from build123d import *

# Parameters (mm, degrees)
F1_DEPTH = 52
F2_DEPTH = 22
F0_R     = 9
F3_DEPTH = 34


with BuildPart() as f1:
    # F0 (on Front) → F1 (new body)
    with BuildSketch(Plane.XZ):
        with BuildLine():
            Line((14, 34), (-54, 34))
            ThreePointArc((-54, 34), (-63.150826, 32.745418), (-71.62633, 29.074258))
            ThreePointArc((-71.62633, 29.074258), (-86.745418, -9.150826), (-54, -34))
            Line((-54, -34), (54, -34))
            ThreePointArc((54, -34), (85.140624, -13.647768), (79, 23.043437))
            ThreePointArc((79, 23.043437), (67.647768, 31.140624), (54, 34))
            Line((54, 34), (27.266499, 34))
            Line((27.266499, 34), (14, 34))
        make_face()
        with BuildLine():
            ThreePointArc((-54, -15), (-69, 0), (-54, 15))
            Line((-54, 15), (54, 15))
            ThreePointArc((54, 15), (69, 0), (54, -15))
            Line((54, -15), (-54, -15))
        make_face(mode=Mode.SUBTRACT)
    extrude(amount=F1_DEPTH)

    # F0 (on Front) → F2 (join)
    with BuildSketch(Plane.XZ):
        with BuildLine():
            ThreePointArc((-71.62633, 29.074258), (-63.150826, 32.745418), (-54, 34))
            Line((-54, 34), (14, 34))
            ThreePointArc((14, 34), (24.606602, 38.393398), (29, 49))
            Line((29, 49), (29, 76))
            ThreePointArc((29, 76), (32.216825, 88.267571), (41.039463, 97.378131))
            Line((41.039463, 97.378131), (-71.62633, 29.074258))
        make_face()
    extrude(amount=F2_DEPTH)

    # F0 (on Front) → F3 (join)
    with BuildSketch(Plane.XZ):
        with BuildLine():
            ThreePointArc((29, 49), (24.606602, 38.393398), (14, 34))
            Line((14, 34), (27.266499, 34))
            Line((27.266499, 34), (54, 34))
            ThreePointArc((54, 34), (67.647768, 31.140624), (79, 23.043437))
            Line((79, 23.043437), (79, 76))
            ThreePointArc((79, 76), (54, 51), (29, 76))
            Line((29, 76), (29, 49))
        make_face()
        with BuildLine():
            ThreePointArc((79, 76), (66.267571, 97.783175), (41.039463, 97.378131))
            ThreePointArc((41.039463, 97.378131), (32.216825, 88.267571), (29, 76))
            ThreePointArc((29, 76), (54, 51), (79, 76))
        make_face()
        with Locations((54, 76)):
            Circle(F0_R, mode=Mode.SUBTRACT)
    extrude(amount=F3_DEPTH)


solid = f1.part
Geometry: final body of the model. Coordinates: model frame, mm. A direction names the side the tool comes from. Coordinates: 2 decimals unless noted, no trailing zeros. Write each loop counter-clockwise with the first axis right and the second up, starting at its lowest first coordinate (ties: lowest second). Pieces come first, ordered by that corner, then holes. Notation, with made-up numbers: (32, 82) - (58, 82) arc R28 cw to (58, 116) - close; hole circle Ø6 at (-16, -28). An arc over 180 degrees is marked (long way). Return JSON: item names as keys, results as strings.
Item 1: Pull-direction query (Z, two-part tool) for faces 5 (the face through (-1, -26, 15)), 6 (the face through (-3, -22, 51)), 7 (the face through (-1, -26, -34)); classes: +Z half, -Z half, draft (parallel to the pull), parting line (faces both ways), or undercut.
Completed:
{"face 5": "undercut", "face 6": "draft", "face 7": "-Z half"}
Item 2: Section query D-D (x = 72.5). Output: boundary loops of the cut face in (y, z), and give its area (3 significant figures).
Completed:
{"outline": "(-52, -28.53) - (0, -28.53) - (0, 92.82) - (-34, 92.82) - (-34, 28.53) - (-52, 28.53) - close", "area": "5,150 mm2"}
Item 3: Pin query (flat end, axial travel): pin 1 Ø17 at (y, z) = (-22, 41) entering from +X; pin 2 Ø9 at (x, y) = (16, -36) entering from +Z; pin 3 Ø10 at (x, y) = (-29, -12) entering from +Z. Return the tip coordinate at first contact, or that it passes through.
Completed:
{"pin 1": "stops at x = 79", "pin 2": "stops at z = 35.27", "pin 3": "stops at z = 57.95"}
Item 4: Line query: L1, parallel to Z at x = 53.5, y = -26.5 (3 decimals); L2, parallel to Z at x = 17, y = -38; L3, parallel to X at y = -26.5, z = 0. Output: solid intervals per line, ascending.
Completed:
{"L1": "z = -34 to -15, 15 to 67.014, 84.986 to 100.995", "L2": "z = -34 to -15, 15 to 34", "L3": "x = -88 to -69, 69 to 88"}
Item 5: Section query B-B (y = -4). Output: boundary loops of the cut face in (x, z).
Completed:
{"outline": "(-71.63, 29.07) arc R34 ccw to (-54, -34) - (54, -34) arc R34 ccw to (79, 23.04) - (79, 76) arc R25 ccw to (41.04, 97.38) - close; hole (-54, -15) - (54, -15) arc R15 ccw to (54, 15) - (-54, 15) arc R15 ccw to start; hole circle Ø18 at (54, 76)"}
Item 6: Section query A-A (z = -9). Output: boundary loops of the cut face in (x, y).
Completed:
{"outline": "(-86.79, -52) - (-66, -52) - (-66, 0) - (-86.79, 0) - close; (66, -52) - (86.79, -52) - (86.79, 0) - (66, 0) - close"}
Item 7: Section query C-C (x = -3). Output: boundary loops of the cut face in (y, z), and give its area (3 significant figures).
Completed:
{"outline": "(-52, -34) - (0, -34) - (0, -15) - (-52, -15) - close; (-52, 15) - (0, 15) - (0, 70.68) - (-22, 70.68) - (-22, 34) - (-52, 34) - close", "area": "2,780 mm2"}
Item 8: Reachability of faces 1 (the face through (18, 0, 34)), 2 (the face through (79, -17, 49)), 3 (the face through (24.72, -27.92, 38.51)), 4 (the face through (-69, -26, 0)) from +Z, -Z, +X, -X, +Y, -Y: full face, straight path, thin tool, end or side. Return the list, or none.
Completed:
{"face 1": "+Z, -Z, +X, -X, +Y", "face 2": "+Z, +X, +Y, -Y", "face 3": "+Z, -X, -Y", "face 4": "+Y, -Y"}
